```python
from build123d import *

# Parameters (mm, degrees)
F0_W      = 101.6
F0_H      = 304.8
F1_DEPTH  = 6.35
F2_R      = 3.175
F3_DEPTH  = 6.35
F4_R      = 14.2875
F5_DEPTH  = 6.35
F6_R      = 14.2875
F7_DEPTH  = 6.35
F8_R      = 2.413
F9_DEPTH  = 6.35
F10_R     = 6.35
F11_DEPTH = 6.35


with BuildPart() as f1:
    # F0 (on Front) → F1 (new body)
    with BuildSketch(Plane.XZ):
        with Locations((102.01661, 91.336442)):
            Rectangle(F0_W, F0_H)
    extrude(amount=F1_DEPTH)

    # F2 (on face) → F3 (cut)
    with BuildSketch(Plane.XZ.offset(6.35)):
        with Locations((102.01661, 215.161442)):
            Circle(F2_R)
    extrude(amount=-F3_DEPTH, mode=Mode.SUBTRACT)

    # F4 (on face) → F5 (cut)
    with BuildSketch(Plane(origin=(0, 0, 0), x_dir=(-1, 0, 0), z_dir=(0, 1, 0))):
        with Locations((-102.01661, -22.455558)):
            Circle(F4_R)
    extrude(amount=-F5_DEPTH, mode=Mode.SUBTRACT)

    # F6 (on face) → F7 (cut)
    with BuildSketch(Plane(origin=(0, 0, 0), x_dir=(-1, 0, 0), z_dir=(0, 1, 0))):
        with Locations((-102.01661, 117.244442)):
            Circle(F6_R)
    extrude(amount=-F7_DEPTH, mode=Mode.SUBTRACT)

    # F8 (on face) → F9 (cut)
    with BuildSketch(Plane(origin=(0, 0, 0), x_dir=(-1, 0, 0), z_dir=(0, 1, 0))):
        with Locations((-84.28741, 136.192842)):
            Circle(F8_R)
        with Locations((-119.74581, 98.296042)):
            Circle(F8_R)
    extrude(amount=-F9_DEPTH, mode=Mode.SUBTRACT)

    # F10 (on face) → F11 (cut)
    with BuildSketch(Plane(origin=(0, 0, 0), x_dir=(-1, 0, 0), z_dir=(0, 1, 0))):
        with Locations((-102.01661, 66.444442)):
            Circle(F10_R)
        with Locations((-102.01661, 169.095919)):
            Circle(F10_R)
    extrude(amount=-F11_DEPTH, mode=Mode.SUBTRACT)


solid = f1.part
```
The listing builds one solid part. Answer for the finished solid, in the listing's coordinates (mm). Round coordinates to 2 decimals unless told otherwise and drop trailing zeros. Order: outer loops, then holes, each group sorted by start corner. A loop starts at its lowest first (then second) coordinate and runs counter-clockwise, first axis right, second up. Notation, with made-up numbers: (7.25, 0) - (55.25, 0) arc R21 cw to (55.25, 27) - close; hole circle Ø5 at (-3.75, 9). An arc over 180 degrees is marked (long way). Put each result on its own line as item: value. Start each with the question number.
(1) Straight lines are drawn through the part: probe 1 along Z at (x, y) = (84, -5.75); probe 2 along Z at (x, y) = (100, -3); probe 3 along Z at (x, y) = (98, -4.75). For each, find the intervals that lie inside material, in ascending order. Write a range as from..to.
(2) Find section B-B (z = 112). Give the vertices of the cut face in (x, y).
(3) Find section C-C (y = -2). State how many separate pieces and enclosed holes the cut face has, plus the area to 3 significant figures.
(4) Find section D-D (z = -25.5). Give the vertices of the cut face in (x, y), plus the area to 3 significant figures.
(5) Find section A-A (x = 102). Give the vertices of the cut face in (y, z), plus the area to 3 significant figures.
(6) Determine the mould class of faces 1 (the flat face through (51.217, -3, 89)), 2 (the cylindrical face through (103.88, -3.13, -8.29)), 3 (the flat face through (101, -3, 243.736)), 4 (the cylindrical face through (95.42, -3.13, 104.57)) for opening direction X: released by +X, released by -X, zero draft, split by the parting line, or undercut.
Reply:
1. probe 1: -61.06..133.8, 138.59..243.74
1. probe 2: -61.06..-36.6, -8.31..60.42, 72.47..103.1, 131.39..163.07, 175.12..212.71, 217.61..243.74
1. probe 3: -61.06..-36.17, -8.74..61.53, 71.36..103.53, 130.96..164.18, 174.01..243.74
2. outline: (51.22, -6.35) - (88.73, -6.35) - (88.73, 0) - (51.22, 0) - close; (115.31, -6.35) - (152.82, -6.35) - (152.82, 0) - (115.31, 0) - close
3. separate pieces: 1
3. enclosed holes: 7
3. area: 29,400 mm^2
4. outline: (51.22, -6.35) - (88.06, -6.35) - (88.06, 0) - (51.22, 0) - close; (115.98, -6.35) - (152.82, -6.35) - (152.82, 0) - (115.98, 0) - close
4. area: 468 mm^2
5. outline: (-6.35, -61.06) - (0, -61.06) - (0, -36.74) - (-6.35, -36.74) - close; (-6.35, -8.17) - (0, -8.17) - (0, 60.09) - (-6.35, 60.09) - close; (-6.35, 72.79) - (0, 72.79) - (0, 102.96) - (-6.35, 102.96) - close; (-6.35, 131.53) - (0, 131.53) - (0, 162.75) - (-6.35, 162.75) - close; (-6.35, 175.45) - (0, 175.45) - (0, 211.99) - (-6.35, 211.99) - close; (-6.35, 218.34) - (0, 218.34) - (0, 243.74) - (-6.35, 243.74) - close
5. area: 1,370 mm^2
6. face 1: released by -X
6. face 2: undercut
6. face 3: zero draft
6. face 4: undercut
